Check sheet for the modelled part. Datum: model origin and axes. Units: mm. A direction names the side the tool comes from. Round coordinates to 2 decimals unless told otherwise and drop trailing zeros. Loops run counter-clockwise (first coordinate to the right, second up) from the corner with the lowest first, then second, coordinate; pieces in that order, holes last. Notation, with made-up numbers: (-4, 46.25) -> (2, 46.25) arc R31 cw to (2, 85.25) -> close; hole circle Ø9 at (-13, -39). An arc over 180 degrees is marked (long way). One line per item, written item: value. Start each with the question number.
1. Go/stop test with flat-tipped pins: pin 1 (5 mm diameter, centred on x = 95.5, z = 57.5, fed in from +Y); pin 2 (1.5 mm diameter, centred on x = 126, z = 6, fed in from -Y); pin 3 (5.5 mm diameter, centred on x = 127, y = -14, fed in from +Z). Record where each tip stops, or that it passes through.
2. Material ranges on L1, parallel to Y at x = 27.5, z = 62; L2, parallel to Y at x = 14, z = 31.5; L3, parallel to X at y = -19.5, z = 14, recorded low to high.
3. Cross-section at D-D on x = 78. Record the cut outline in (y, z), then the cut area to 3 significant figures.
4. Cross-section at B-B on x = 10. Record the cut outline in (y, z), then the cut area to 3 significant figures.
5. Set-up check for faces 4 (the face through (7, -25, 2)), 5 (the face through (126, -16, 2)), 6 (the face through (3.11, 1.01, 90.44)), 7 (the face through (128.669, -2.493, 7.026)): record each of +Z, -Z, +X, -X, +Y, -Y from which the full face is reachable in a straight line by a thin tool's end or side.
6. Cross-section at A-A on z = 6.5. Record the cut outline in (x, y).
7. Release check for a two-part mould opening along Z. For faces 1 (the face through (128.669, 1.014, 7.026)), 2 (the face through (4, -3, 92)), 3 (the face through (127, -3, 7)) record: +Z half, -Z half, draft (parallel to the pull), parting line (faces both ways), or undercut.
8. Cross-section at C-C on y = -25. Record the cut outline in (x, z), then the cut area to 3 significant figures.
from build123d import *

# Parameters (mm, degrees)
SKETCH_W          = 129
SKETCH_H          = 97
PAD_DEPTH         = 30
BOX_W             = 15
BOX_H             = 95
BOX_DEPTH         = 10
BOX001_W          = 15
BOX001_H          = 11
BOX001_DEPTH      = 28
BOX002_W          = 5
BOX002_H          = 10
BOX002_DEPTH      = 28
BOX003_W          = 5
BOX003_H          = 85
BOX003_DEPTH      = 20
CYLINDER_R        = 1.75
CYLINDER_DEPTH    = 5
CYLINDER001_R     = 1.75
CYLINDER001_DEPTH = 5
CYLINDER002_R     = 1.75
CYLINDER002_DEPTH = 5
CYLINDER003_R     = 1.75
CYLINDER003_DEPTH = 5


with BuildPart() as part:
    # Sketch → Pad (new body)
    with BuildSketch(Plane.XZ):
        with Locations((64.5, 48.5)):
            Rectangle(SKETCH_W, SKETCH_H)
    extrude(amount=PAD_DEPTH)

    # Box → Box (cut)
    with BuildSketch(Plane(origin=(0, -20, 2), x_dir=(1, 0, 0), z_dir=(0, -1, 0))):
        with Locations((7.5, 47.5)):
            Rectangle(BOX_W, BOX_H)
    extrude(amount=BOX_DEPTH, mode=Mode.SUBTRACT)

    # Box001 → Box001 (cut)
    with BuildSketch(Plane(origin=(0, -2, 86), x_dir=(1, 0, 0), z_dir=(0, -1, 0))):
        with Locations((7.5, 5.5)):
            Rectangle(BOX001_W, BOX001_H)
    extrude(amount=BOX001_DEPTH, mode=Mode.SUBTRACT)

    # Box002 → Box002 (cut)
    with BuildSketch(Plane(origin=(124, -2, 2), x_dir=(1, 0, 0), z_dir=(0, -1, 0))):
        with Locations((2.5, 5)):
            Rectangle(BOX002_W, BOX002_H)
    extrude(amount=BOX002_DEPTH, mode=Mode.SUBTRACT)

    # Box003 → Box003 (cut)
    with BuildSketch(Plane(origin=(124, -10, 12), x_dir=(1, 0, 0), z_dir=(0, -1, 0))):
        with Locations((2.5, 42.5)):
            Rectangle(BOX003_W, BOX003_H)
    extrude(amount=BOX003_DEPTH, mode=Mode.SUBTRACT)

    # Cylinder → Cylinder (join)
    with BuildSketch(Plane(origin=(127, 2, 6.5), x_dir=(1, 0, 0), z_dir=(0, -1, 0))):
        Circle(CYLINDER_R)
    extrude(amount=CYLINDER_DEPTH)

    # Cylinder001 → Cylinder001 (join)
    with BuildSketch(Plane(origin=(4.5, 2, 91.5), x_dir=(1, 0, 0), z_dir=(0, -1, 0))):
        Circle(CYLINDER001_R)
    extrude(amount=CYLINDER001_DEPTH)

    # Cylinder002 → Cylinder002 (join)
    with BuildSketch(Plane(origin=(78, 2, 34), x_dir=(1, 0, 0), z_dir=(0, -1, 0))):
        Circle(CYLINDER002_R)
    extrude(amount=CYLINDER002_DEPTH)

    # Cylinder003 → Cylinder003 (join)
    with BuildSketch(Plane(origin=(78, 2, 67), x_dir=(1, 0, 0), z_dir=(0, -1, 0))):
        Circle(CYLINDER003_R)
    extrude(amount=CYLINDER003_DEPTH)


solid = part.part
Taken from the geometry:
1. pin 1: stops at y = 0
1. pin 2: stops at y = -3
1. pin 3: stops at z = 2
2. L1: y = -30 to 0
2. L2: y = -20 to 0
2. L3: x = 0 to 124
3. outline: (-30, 0) -> (0, 0) -> (0, 32.25) -> (2, 32.25) -> (2, 35.75) -> (0, 35.75) -> (0, 65.25) -> (2, 65.25) -> (2, 68.75) -> (0, 68.75) -> (0, 97) -> (-30, 97) -> close
3. area: 2,920 mm2
4. outline: (-30, 0) -> (0, 0) -> (0, 97) -> (-2, 97) -> (-2, 86) -> (-20, 86) -> (-20, 2) -> (-30, 2) -> close
4. area: 1,760 mm2
5. face 4: +Z, -X, -Y
5. face 5: +X, -Y
5. face 6: +Y
5. face 7: -Y
6. outline: (0, -20) -> (15, -20) -> (15, -30) -> (124, -30) -> (124, -2) -> (125.25, -2) -> (125.25, -3) -> (128.75, -3) -> (128.75, -2) -> (129, -2) -> (129, 0) -> (128.75, 0) -> (128.75, 2) -> (125.25, 2) -> (125.25, 0) -> (0, 0) -> close
7. face 1: parting line
7. face 2: draft
7. face 3: undercut
8. outline: (0, 0) -> (129, 0) -> (129, 2) -> (124, 2) -> (124, 97) -> (15, 97) -> (15, 2) -> (0, 2) -> close
8. area: 10,600 mm2
